CAD build for the part. Positions are in the model's coordinates, mm. A direction names the side the tool comes from. Give positions to 0.01 mm unless a question says otherwise; leave off trailing zeros. Loops run counter-clockwise (first coordinate to the right, second up) from the corner with the lowest first, then second, coordinate; pieces in that order, holes last. Notation, with made-up numbers: (41, 54.5) -> (76, 54.5) arc R26 cw to (76, 82.5) -> close; hole circle Ø9 at (34, 68.5). An arc over 180 degrees is marked (long way). Write each question's results on one line, items separated by ' | '. Start each with the question number.
```python
from build123d import *

# Parameters (mm, degrees)
BOSS_EXTRUDE1_DEPTH      = 29.21
SKETCH2_R                = 3.175
BOSS_EXTRUDE2_DEPTH      = 3.81
BOSS_EXTRUDE3_START      = -3.81
SKETCH3_R                = 3.175
SKETCH3_R_2              = 3.181823626
BOSS_EXTRUDE3_DEPTH      = 3.81
BOSS_EXTRUDE4_DEPTH      = 1.524
BOSS_EXTRUDE4_DEPTH_BACK = 3.302
SKETCH4_R                = 3.109705259
SKETCH4_R_2              = 2.977374329


with BuildPart() as part:
    # Sketch1 → Boss-Extrude1 (new body)
    with BuildSketch(Plane.XY):
        with BuildLine():
            Line((-445.741932109, 248.343634647), (-445.112071681, 252.347923806))
            Line((-445.112071681, 252.347923806), (-457.363663126, 254.275055523))
            Line((-457.363663126, 254.275055523), (-458.927145779, 254.520985778))
            ThreePointArc((-458.927145779, 254.520985778), (-462.17729329, 255.913510824), (-464.467858916, 258.607187485))
            ThreePointArc((-464.467858916, 258.607187485), (-465.308453245, 262.469514201), (-464.120754615, 266.239598875))
            ThreePointArc((-464.120754615, 266.239598875), (-463.399050509, 268.135245999), (-463.477224231, 270.162121354))
            ThreePointArc((-463.477224231, 270.162121354), (-463.334265537, 274.465295187), (-460.978145391, 278.068965549))
            Line((-460.978145391, 278.068965549), (-467.519631336, 279.097918))
            Line((-467.519631336, 279.097918), (-471.71455165, 252.429035234))
            Line((-471.71455165, 252.429035234), (-445.741932109, 248.343634647))
        make_face()
    extrude(amount=-BOSS_EXTRUDE1_DEPTH)

    # Sketch2 → Boss-Extrude2 (add)
    with BuildSketch(Plane.XY):
        Polygon((-467.519631336, 279.097918), (-471.71455165, 252.429035234), (-445.741932109, 248.343634647), (-441.565787186, 274.887665754), align=None)
        with Locations((-455.996603091, 271.987703521)):
            Circle(SKETCH2_R, mode=Mode.SUBTRACT)
        with Locations((-457.615851502, 262.119672583)):
            Circle(SKETCH2_R, mode=Mode.SUBTRACT)
    extrude(amount=BOSS_EXTRUDE2_DEPTH)

    # Sketch3 → Boss-Extrude3 (add)
    with BuildSketch(Plane(origin=(0, 0, -29.21), x_dir=(-1, 0, 0), z_dir=(0, 0, -1)).offset(BOSS_EXTRUDE3_START)):
        with BuildLine():
            Line((460.978145391, 278.068965549), (441.565787186, 274.887665754))
            Line((441.565787186, 274.887665754), (445.112071681, 252.347923806))
            Line((445.112071681, 252.347923806), (458.927145779, 254.520985778))
            ThreePointArc((458.927145779, 254.520985778), (464.657191184, 258.991661442), (464.120754615, 266.239598875))
            ThreePointArc((464.120754615, 266.239598875), (463.399050509, 268.135245999), (463.477224231, 270.162121354))
            ThreePointArc((463.477224231, 270.162121354), (463.334265537, 274.465295187), (460.978145391, 278.068965549))
        make_face()
        with Locations(Location((455.996603091, 271.987703521, 0), (0, 0, 180))):
            Circle(SKETCH3_R, mode=Mode.SUBTRACT)
        with Locations((457.611982645, 262.114049476)):
            Circle(SKETCH3_R_2, mode=Mode.SUBTRACT)
    extrude(amount=BOSS_EXTRUDE3_DEPTH)

    # Sketch4 → Boss-Extrude4 (add, two sides: drawn at the far end of the back side and taken through both)
    with BuildSketch(Plane(origin=(2.279673246, 246.113529363, 11.60731603), x_dir=(0.9999571992457364, -0.009241736857419818, -0.0004358629151659602), z_dir=(0.009252009328930062, 0.998846950490518, 0.04710806533037038)).offset(-BOSS_EXTRUDE4_DEPTH_BACK)):
        Polygon((-448.019641178, 7.893719141), (-448.019641178, -18.159221947), (-474.014513074, -18.159221947), (-474.028905268, 8.086182696), (-474.014513074, 41.069520713), (-483.533549488, 62.101622956), (-458.002958068, 64.465529415), (-448.005248984, 40.877057158), align=None)
        with Locations(Location((-465.863593213, 52.113287489, 0), (0, 0, 270))):
            Circle(SKETCH4_R, mode=Mode.SUBTRACT)
        with Locations(Location((-461.180575409, -5.817624253, 0), (0, 0, 270))):
            Circle(SKETCH4_R_2, mode=Mode.SUBTRACT)
    extrude(amount=BOSS_EXTRUDE4_DEPTH + BOSS_EXTRUDE4_DEPTH_BACK)


solid = part.part
```
Q1. Saw through at C-C, the plane z = -16. List the corners of the cut face in (x, y), then the cut area to 3 significant figures.
Q2. Mould opens along X. For faces 3 (the face through (-443.683, 261.43, 1.878)), 4 (the face through (-453, 265, -25.4)), 5 (the face through (-460.788, 262.259, 1.878)) say: pulls with the +X half, pulls with the -X half, needs draft (parallel to the pull), parting line crosses it, or undercut.
Q3. Saw through at B-B, the plane x = -448.5. List the corners of the cut face in (y, z).
Q4. Which spindle directions (+Z, -Z, +X, -X, +Y, -Y) get a long thin tool onto all of the face, cutting with end or side? Do faces 1 (the face through (-468.656, 252.525, -51.428)), 2 (the face through (-465.31, 262.41, -12.52)). Say none if no direction does.
Q5. Wall check: L1, parallel to Z at x = -451, y = 275; L2, parallel to Y at x = -464, z = -19.5; L3, parallel to Z at x = -469, y = 265.5. Give the ranges that are in metal, low to high.
Q6. Saw through at D-D, the plane y = 276.5. List the corners of the cut face in (x, z).
Q7. Drop flat-ended pins along their axis: pin 1 (12 mm diameter, centred on x = -460, y = 267.5, fed in from +Z); pin 2 (3 mm diameter, centred on x = -471.5, z = 19.5, fed in from -Y); pin 3 (8 mm diameter, centred on x = -458, z = -37.5, fed in from -Y). Give the stop position or say it passes through.
Q8. Saw through at A-A, the plane y = 273. List the corners of the cut face in (x, z), then the cut area to 3 significant figures.
Answer block:
1) outline: (-471.75, 248.5) -> (-445.74, 248.26) -> (-445.74, 248.34) -> (-445.11, 252.35) -> (-445.7, 252.44) -> (-445.7, 253.09) -> (-450.09, 253.13) -> (-458.93, 254.52) arc R7.73 cw to (-464.47, 258.61) arc R7.7 cw to (-464.12, 266.24) arc R5.08 ccw to (-463.48, 270.16) arc R7.99 cw to (-460.98, 278.07) -> (-467.52, 279.1) -> (-471.57, 253.33) -> (-471.71, 253.33) -> close | area: 290 mm2
2) face 3: pulls with the +X half | face 4: needs draft | face 5: undercut
3) outline: (246.13, 29.79) -> (248.78, -26.44) -> (248.78, -29.21) -> (248.91, -29.21) -> (249.21, -35.7) -> (254.04, -35.57) -> (253.74, -29.21) -> (276.02, -29.21) -> (276.02, -25.4) -> (253.56, -25.4) -> (252.88, -11) -> (252.88, 0) -> (276.01, 0) -> (276.01, 3.81) -> (252.18, 3.81) -> (250.95, 30.01) -> close
4) face 1: -Z, -X, +Y | face 2: +X
5) L1: z = -29.21 to -25.4, 0 to 3.81 | L2: y = 248.59 to 257.82, 266.44 to 278.54 | L3: z = -29.21 to 3.81
6) outline: (-467.93, -29.21) -> (-451.4, -29.21) -> (-451.4, -25.4) -> (-462.36, -25.4) -> (-462.36, 0) -> (-451.5, 0) -> (-451.5, 3.81) -> (-467.93, 3.81) -> close
7) pin 1: stops at z = 3.81 | pin 2: stops at y = 246.75 | pin 3: stops at y = 249.19
8) outline: (-468.48, -29.21) -> (-459.01, -29.21) -> (-459.01, -25.4) -> (-463.65, -25.4) -> (-463.65, 0) -> (-459.01, 0) -> (-459.01, 3.81) -> (-468.48, 3.81) -> close; (-452.99, -29.21) -> (-441.86, -29.21) -> (-441.86, -25.4) -> (-452.99, -25.4) -> close; (-452.99, 0) -> (-441.86, 0) -> (-441.86, 3.81) -> (-452.99, 3.81) -> close | area: 280 mm2
